Read the model definition and answer for the solid it produces. Units are mm, in the model's axes. A direction names the side the tool comes from. Round coordinates to 2 decimals unless told otherwise and drop trailing zeros. Order: outer loops, then holes, each group sorted by start corner. A loop starts at its lowest first (then second) coordinate and runs counter-clockwise, first axis right, second up. Notation, with made-up numbers: (32.25, 11.5) - (41.25, 11.5) arc R20 ccw to (41.25, 17.5) - close; hole circle Ø8 at (65.5, 63.25). An arc over 180 degrees is marked (long way). One line per question, with ' | ' between items. Start each with the question number.
1) The part is cut by section D-D, the plane x = 11. Give the vertices of the cut face in (y, z), plus the area to 3 significant figures.
2) The part is cut by section B-B, the plane x = 38. Give the vertices of the cut face in (y, z), plus the area to 3 significant figures.
3) Straight lines are drawn through the part: line 1 (Z direction, x = 71.5, y = 1.3); line 2 (Z direction, x = 53, y = 2.7); line 3 (X direction, y = 0.4, z = -16.5). For each, find the intervals that lie inside material, in ascending order. Write a range as from..to.
4) The part is cut by section C-C, the plane y = 1.3. Count the separate pieces of the cut face and the enclosed holes in it, plus the area to 3 significant figures.
5) The part is cut by section A-A, the plane z = -28. Give the vertices of the cut face in (x, y), plus the area to 3 significant figures.
6) The mould has two halves that part along Z. Classify faces 6 (the flat face through (4, 2, -30)), 7 (the flat face through (46, 2, -4)), 8 (the flat face through (38, 2, -42)): pulls with the +Z half, pulls with the -Z half, needs draft (parallel to the pull), parting line crosses it, or undercut.
7) For faces 1 (the flat face through (17.5, 2, -2)), 2 (the flat face through (73, 2, -25)), 3 (the flat face through (2, 2, -8)), 4 (the flat face through (25.5, 2, -40)), 5 (the flat face through (0, 2, -38)), determine the directions among +Z, -Z, +X, -X, +Y, -Y from which every point of the face is accessible in a straight line to the end or side of a thin tool.
8) Flat-ended cylindrical pins translate along their axes: pin 1 (2 mm diameter, centred on x = 31, y = 2.5, fed in from -Z); pin 2 (1.5 mm diameter, centred on x = 13.5, y = 3, fed in from +Z); pin 3 (2 mm diameter, centred on y = 2, z = -12, fed in from -X). Find the tip coordinate at first contact, or state that the pin passes through.
Autodesk Inventor part; units mm, degrees
ref_plane "YZ Plane" through (0, 0, 0) normal (1, 0, 0) x (0, 1, 0)
ref_plane "XZ Plane" through (0, 0, 0) normal (0, 1, 0) x (-1, 0, 0)
ref_plane "XY Plane" through (0, 0, 0) normal (0, 0, 1) x (1, 0, 0)
sketch "Sketch1" plane through (0, 0, 0) normal (0, 1, 0) x (-1, 0, 0)
  line L0 (0, 0) -> (-75, 0)
  line L1 (-75, 0) -> (-75, -42)
  line L2 (-75, -42) -> (0, -42)
  line L3 (0, -42) -> (0, 0)
  line L4 (-8, -18) -> (-28, -18)
  line L5 (-28, -18) -> (-28, -12)
  line L6 (-28, -12) -> (-8, -12)
  line L7 (-8, -12) -> (-8, -18)
  circle A0 centre (-38, -28) radius 3.5
  circle A1 centre (-53, -28) radius 3.5
  dimension "d0" = 75
  dimension "d1" = 42
  dimension "d2" = 20
  dimension "d3" = 6
  dimension "d4" = 12
  dimension "d5" = 8
  dimension "d6" = 7
  dimension "d7" = 28
  dimension "d8" = 38
  dimension "d9" = 15
extrude "Extrusion1" add sketch "Sketch1" along normal blind 4
sketch "Sketch2" plane through (0, 4, 0) normal (0, 1, 0) x (1, 0, 0)
  line L0 (0, 42) -> (0, 0) construction
  line L1 (75, 42) -> (0, 42) construction
  line L2 (75, 0) -> (75, 42) construction
  line L3 (0, 0) -> (75, 0) construction
  line L4 (4, 38) -> (4, 4) construction
  line L5 (4, 4) -> (71, 4) construction
  line L6 (71, 4) -> (71, 38) construction
  line L7 (71, 38) -> (4, 38) construction
  line L8 (0, 42) -> (0, 0) construction
  line L9 (0, 21) -> (75, 21) construction
  line L10 (37.5, 42) -> (37.5, 0) construction
  line L11 (0, 34) -> (4, 34)
  line L12 (4, 34) -> (4, 25)
  line L13 (4, 25) -> (0, 25)
  line L14 (0, 25) -> (0, 34)
  line L15 (75, 42) -> (0, 42)
  line L16 (9.5, 38) -> (17.5, 38)
  line L17 (17.5, 38) -> (17.5, 42)
  line L18 (17.5, 42) -> (9.5, 42)
  line L19 (9.5, 42) -> (9.5, 38)
  line L20 (25.5, 38) -> (33.5, 38)
  line L21 (33.5, 38) -> (33.5, 42)
  line L22 (33.5, 42) -> (25.5, 42)
  line L23 (25.5, 42) -> (25.5, 38)
  line L24 (75, 34) -> (71, 34)
  line L25 (71, 34) -> (71, 25)
  line L26 (71, 25) -> (75, 25)
  line L27 (75, 25) -> (75, 34)
  line L28 (65.5, 38) -> (57.5, 38)
  line L29 (57.5, 38) -> (57.5, 42)
  line L30 (57.5, 42) -> (65.5, 42)
  line L31 (65.5, 42) -> (65.5, 38)
  line L32 (49.5, 38) -> (41.5, 38)
  line L33 (41.5, 38) -> (41.5, 42)
  line L34 (41.5, 42) -> (49.5, 42)
  line L35 (49.5, 42) -> (49.5, 38)
  line L36 (75, 0) -> (0, 0) construction
  line L37 (71, 4) -> (4, 4) construction
  line L38 (0, 8) -> (4, 8)
  line L39 (4, 8) -> (4, 17)
  line L40 (4, 17) -> (0, 17)
  line L41 (0, 17) -> (0, 8)
  line L42 (75, 0) -> (0, 0)
  line L43 (9.5, 4) -> (17.5, 4)
  line L44 (17.5, 4) -> (17.5, 0)
  line L45 (17.5, 0) -> (9.5, 0)
  line L46 (9.5, 0) -> (9.5, 4)
  line L47 (25.5, 4) -> (33.5, 4)
  line L48 (33.5, 4) -> (33.5, 0)
  line L49 (33.5, 0) -> (25.5, 0)
  line L50 (25.5, 0) -> (25.5, 4)
  line L51 (49.5, 4) -> (41.5, 4)
  line L52 (49.5, 0) -> (49.5, 4)
  line L53 (41.5, 0) -> (49.5, 0)
  line L54 (41.5, 4) -> (41.5, 0)
  line L55 (57.5, 4) -> (57.5, 0)
  line L56 (65.5, 4) -> (57.5, 4)
  line L57 (57.5, 0) -> (65.5, 0)
  line L58 (71, 8) -> (71, 17)
  line L59 (71, 17) -> (75, 17)
  line L60 (75, 17) -> (75, 8)
  line L61 (75, 8) -> (71, 8)
  line L62 (65.5, 0) -> (65.5, 4)
  dimension "d12" = 4
  dimension "d13" = 4
  dimension "d14" = 8
  dimension "d15" = 8
  dimension "d16" = 8
  dimension "d17" = 8
  dimension "d18" = 4
extrude "Extrusion2" cut sketch "Sketch2" against normal up to surface (4 mm away)
properties part number "left" material "PBT Plastic Black"
Values:
1) outline: (0, -38) - (4, -38) - (4, -18) - (0, -18) - close; (0, -12) - (4, -12) - (4, -4) - (0, -4) - close | area: 112 mm^2
2) outline: (0, -42) - (4, -42) - (4, -31.5) - (0, -31.5) - close; (0, -24.5) - (4, -24.5) - (4, 0) - (0, 0) - close | area: 140 mm^2
3) line 1: z = -42..-34, -25..-17, -8..0 | line 2: z = -42..-31.5, -24.5..0 | line 3: x = 4..8, 28..71
4) separate pieces: 1 | enclosed holes: 3 | area: 2,550 mm^2
5) outline: (4, 0) - (34.5, 0) - (34.5, 4) - (4, 4) - close; (41.5, 0) - (49.5, 0) - (49.5, 4) - (41.5, 4) - close; (56.5, 0) - (71, 0) - (71, 4) - (56.5, 4) - close | area: 212 mm^2
6) face 6: undercut | face 7: pulls with the +Z half | face 8: pulls with the -Z half
7) face 1: +Z, +Y, -Y | face 2: +X, +Y, -Y | face 3: -X, +Y, -Y | face 4: -Z, +Y, -Y | face 5: +Z, -Z, -X, +Y, -Y
8) pin 1: stops at z = -38 | pin 2: stops at z = -4 | pin 3: stops at x = 4
